from build123d import *

# Parameters (mm, degrees)
SKETCH_W     = 6
SKETCH_H     = 6
PAD_DEPTH    = 3
SKETCH001_R  = 1.75
PAD001_DEPTH = 1.2
SKETCH002_W  = 0.2
SKETCH002_H  = 0.7
PAD002_DEPTH = 1


with BuildPart() as part:
    # Sketch → Pad (new body)
    with BuildSketch(Plane.XY):
        Rectangle(SKETCH_W, SKETCH_H)
    extrude(amount=PAD_DEPTH)

    # Sketch001 (on Face6 of Pad) → Pad001 (join)
    with BuildSketch(Plane.XY.offset(3)):
        Circle(SKETCH001_R)
    extrude(amount=PAD001_DEPTH)

    # Sketch002 (on Face4 of Pad001) → Pad002 (join, symmetric)
    with BuildSketch(Plane(origin=(0, 0, 0), x_dir=(1, 0, 0), z_dir=(0, 0, -1))):
        with Locations((-3.1, 1.85)):
            Rectangle(SKETCH002_W, SKETCH002_H)
        with Locations((-3.1, -1.85)):
            Rectangle(SKETCH002_W, SKETCH002_H)
    pad002 = extrude(amount=PAD002_DEPTH, both=True)

    # Mirrored: Pad002 across YZ
    add(pad002.mirror(Plane.YZ))


solid = part.part
Source: CAD feature listing. Evaluate the final solid. Frame: model axes, mm. A direction names the side the tool comes from. Give positions to 0.01 mm unless a question says otherwise; leave off trailing zeros. Write each loop counter-clockwise with the first axis right and the second up, starting at its lowest first coordinate (ties: lowest second). Pieces come first, ordered by that corner, then holes. Notation, with made-up numbers: M -38,74.25 L -22,74.25 A16 ccw -22,86.25 Z; hole C 21,-11 d2. An arc over 180 degrees is marked long. Return JSON: item names as keys, results as strings. Group by question number.
1) Cut plane A-A, the plane z = -0.1. Output: boundary loops of the cut face in (x, y), plus the area to 3 significant figures.
2) Pull-direction query (X, two-part tool) for faces 3 (the face through (0, 0, 4.2)), 4 (the face through (1.617, -0.67, 3.592)), 5 (the face through (0, 0, 0)); classes: pulls with the +X half, pulls with the -X half, needs draft (parallel to the pull), parting line crosses it, or undercut.
3) Set-up query: faces 1 (the face through (0, -3, 1)), 2 (the face through (1.3, 1.4, 3)). Return all of +Z, -Z, +X, -X, +Y, -Y with unobstructed straight access to the full face (end or side cutting, diameter ignored); none if empty.
4) Pin query (flat end, axial travel): P1, Ø1.5, axis at y = 0.5, z = 1.5, coming from the +X side; P2, Ø3, axis at x = -1.5, y = -1, coming from the +Z side; P3, Ø1.8, axis at x = -1.5, y = 1.5, coming from the -Z side. Return the tip coordinate at first contact, or that it passes through.
5) Material intervals for line 1 along X through (y, z) = (-1, 0.9); line 2 along Z through (x, y) = (1, 2.2); line 3 along Y through (x, z) = (0.75, 3.8), sorted ascending. Write a range as [from, to].
6) Cut plane C-C, the plane x = 0. Output: boundary loops of the cut face in (y, z).
7) Cut plane B-B, the plane z = 0.6. Output: boundary loops of the cut face in (x, y), plus the area to 3 significant figures.
Recorded:
{
 "1": {"outline": "M -3.2,-2.2 L -3,-2.2 L -3,-1.5 L -3.2,-1.5 Z; M -3.2,1.5 L -3,1.5 L -3,2.2 L -3.2,2.2 Z; M 3,-2.2 L 3.2,-2.2 L 3.2,-1.5 L 3,-1.5 Z; M 3,1.5 L 3.2,1.5 L 3.2,2.2 L 3,2.2 Z", "area": "0.560 mm²"},
 "2": {"face 3": "needs draft", "face 4": "parting line crosses it", "face 5": "undercut"},
 "3": {"face 1": "+Z, -Z, +X, -X, -Y", "face 2": "+Z"},
 "4": {"P1": "stops at x = 3", "P2": "stops at z = 4.2", "P3": "stops at z = 0"},
 "5": {"line 1": "x = [-3, 3]", "line 2": "z = [0, 3]", "line 3": "y = [-1.58, 1.58]"},
 "6": {"outline": "M -3,0 L 3,0 L 3,3 L 1.75,3 L 1.75,4.2 L -1.75,4.2 L -1.75,3 L -3,3 Z"},
 "7": {"outline": "M -3.2,-2.2 L -3,-2.2 L -3,-3 L 3,-3 L 3,-2.2 L 3.2,-2.2 L 3.2,-1.5 L 3,-1.5 L 3,1.5 L 3.2,1.5 L 3.2,2.2 L 3,2.2 L 3,3 L -3,3 L -3,2.2 L -3.2,2.2 L -3.2,1.5 L -3,1.5 L -3,-1.5 L -3.2,-1.5 Z", "area": "36.6 mm²"}
}
